Verification items for the finished model (mm, model axes). A direction names the side the tool comes from. Coordinates: 2 decimals unless noted, no trailing zeros. Order: outer loops, then holes, each group sorted by start corner. A loop starts at its lowest first (then second) coordinate and runs counter-clockwise, first axis right, second up. Notation, with made-up numbers: (1.5, -20) -> (27.5, -20) arc R18 ccw to (27.5, -6) -> close; hole circle Ø1 at (37.5, 76.25). An arc over 180 degrees is marked (long way). Write each question's results on one line, items separated by ' | '. Start each with the question number.
(1) Set-up check for faces 4 (the cylindrical face through (0.9, 0.86, -25.35)), 5 (the flat face through (24, 3, -6)): record each of +Z, -Z, +X, -X, +Y, -Y from which the full face is reachable in a straight line by a thin tool's end or side.
(2) Go/stop test with flat-tipped pins: pin 1 (0.7 mm diameter, centred on x = 23.5, y = 3, fed in from +Z); pin 2 (1 mm diameter, centred on x = 24.5, z = -31.5, fed in from -Y); pin 3 (4.5 mm diameter, centred on x = 10.5, y = 10, fed in from +Z). Record where each tip stops, or that it passes through.
(3) Cross-section at D-D on x = 2.5. Enter the section's corners in (y, z).
(4) Cross-section at A-A on z = -33. Enter the section's corners in (x, y), and give its area (3 significant figures).
(5) Cross-section at B-B on y = 14.5. Enter the section's corners in (x, z).
(6) Draft check along Y on faces 1 (the flat face through (14, 11, -48)), 2 (the flat face through (27, 10, -25)), 3 (the flat face through (13, 0, -25)). Enter one of: +Y half, -Y half, draft (parallel to the pull), parting line (faces both ways), or undercut.
(7) Thickness scan on probe 1 along Y at (x, z) = (24, -2.1); probe 2 along X at (y, z) = (16.75, -21.5); probe 3 along Y at (x, z) = (17, -42). Record the ranges inside material, lowest first. Write a range as [from, to].
(8) Cross-section at C-C on x = 6.5. Enter the section's corners in (y, z).
```python
from build123d import *

# Parameters (mm, degrees)
SKETCH1_W               = 27
SKETCH1_H               = 20
BOSS_EXTRUDE1_DEPTH     = 50
SKETCH2_W               = 19
SKETCH2_H               = 14
BOSS_EXTRUDE2_DEPTH     = 2
SKETCH3_W               = 23
SKETCH3_H               = 2
CUT_EXTRUDE1_DEPTH      = 48
SKETCH4_W               = 0.5
SKETCH4_H               = 9
SKETCH4_W_2             = 19
SKETCH4_H_2             = 0.5
BOSS_EXTRUDE3_DEPTH     = 48
FILLET1_R               = 3
SKETCH6_R               = 1.1
CUT_EXTRUDE2_DEPTH      = 6
CUT_EXTRUDE3_DEPTH      = 61.241181927
CUT_EXTRUDE3_DEPTH_BACK = 48
SKETCH14_W              = 19
SKETCH14_H              = 1.5


with BuildPart() as part:
    # Sketch1 → Boss-Extrude1 (new body)
    with BuildSketch(Plane.XY):
        with Locations((13.5, 10)):
            Rectangle(SKETCH1_W, SKETCH1_H)
        Polygon((4, 17), (23, 17), (23, 16), (23, 4), (23, 3), (4, 3), (4, 4), (4, 16), align=None, mode=Mode.SUBTRACT)
    extrude(amount=-BOSS_EXTRUDE1_DEPTH)

    # Sketch2 → Boss-Extrude2 (add)
    with BuildSketch(Plane(origin=(0, 0, -50), x_dir=(-1, 0, 0), z_dir=(0, 0, -1))):
        with Locations((-13.5, 10)):
            Rectangle(SKETCH2_W, SKETCH2_H)
    extrude(amount=-BOSS_EXTRUDE2_DEPTH)

    # Sketch3 → Cut-Extrude1 (cut)
    with BuildSketch(Plane.XY):
        with Locations((13.5, 13)):
            Rectangle(SKETCH3_W, SKETCH3_H)
    extrude(amount=-CUT_EXTRUDE1_DEPTH, mode=Mode.SUBTRACT)

    # Sketch4 → Boss-Extrude3 (add)
    with BuildSketch(Plane.XY):
        with Locations((4.25, 7.5)):
            Rectangle(SKETCH4_W, SKETCH4_H)
        with Locations((22.75, 7.5)):
            Rectangle(SKETCH4_W, SKETCH4_H)
        with Locations((13.5, 16.75)):
            Rectangle(SKETCH4_W_2, SKETCH4_H_2)
    extrude(amount=-BOSS_EXTRUDE3_DEPTH)

    # Fillet1
    fillet1_edges = [part.edges().sort_by_distance(p)[0] for p in [
        (0, 0, -25),
        (0, 20, -25),
        (27, 20, -25),
        (27, 0, -25),
    ]]
    fillet(fillet1_edges, radius=FILLET1_R)

    # Sketch6 → Cut-Extrude2 (cut)
    with BuildSketch(Plane.XY):
        with Locations((3, 17)):
            Circle(SKETCH6_R)
        with Locations((24, 17)):
            Circle(SKETCH6_R)
        with Locations((24, 3)):
            Circle(SKETCH6_R)
        with Locations((3, 3)):
            Circle(SKETCH6_R)
    extrude(amount=-CUT_EXTRUDE2_DEPTH, mode=Mode.SUBTRACT)

    # Sketch14 → Cut-Extrude3 (cut, two sides: drawn at the far end of the back side and taken through both)
    with BuildSketch(Plane.XY.offset(-CUT_EXTRUDE3_DEPTH_BACK)):
        with Locations((13.5, 17.25)):
            Rectangle(SKETCH14_W, SKETCH14_H)
    extrude(amount=CUT_EXTRUDE3_DEPTH + CUT_EXTRUDE3_DEPTH_BACK, mode=Mode.SUBTRACT)


solid = part.part
```
Results are:
1) face 4: +Z, -Z, -X, -Y | face 5: +Z
2) pin 1: stops at z = -6 | pin 2: stops at y = 0 | pin 3: stops at z = -48
3) outline: (0.04, -50) -> (19.96, -50) -> (19.96, 0) -> (17.98, 0) -> (17.98, -6) -> (16.02, -6) -> (16.02, 0) -> (14, 0) -> (14, -48) -> (12, -48) -> (12, 0) -> (3.98, 0) -> (3.98, -6) -> (2.02, -6) -> (2.02, 0) -> (0.04, 0) -> close
4) outline: (0, 3) arc R3 ccw to (3, 0) -> (24, 0) arc R3 ccw to (27, 3) -> (27, 17) arc R3 ccw to (24, 20) -> (3, 20) arc R3 ccw to (0, 17) -> close; hole (2, 12) -> (4.5, 12) -> (4.5, 3) -> (22.5, 3) -> (22.5, 12) -> (25, 12) -> (25, 14) -> (23, 14) -> (23, 18) -> (4, 18) -> (4, 14) -> (2, 14) -> close | area: 248 mm2
5) outline: (0, -50) -> (27, -50) -> (27, 0) -> (23, 0) -> (23, -48) -> (4, -48) -> (4, 0) -> (0, 0) -> close
6) face 1: undercut | face 2: draft | face 3: -Y half
7) probe 1: y = [0, 1.9], [4.1, 12], [14, 15.9], [18.1, 20] | probe 2: x = [0, 4], [23, 27] | probe 3: y = [0, 3], [18, 20]
8) outline: (0, -50) -> (20, -50) -> (20, 0) -> (18, 0) -> (18, -48) -> (3, -48) -> (3, 0) -> (0, 0) -> close
